Work out the finished part from the listing and answer in its coordinate system (mm). Face numbers are marked on the shaded views. A direction names the side the tool comes from. Round coordinates to 2 decimals unless told otherwise and drop trailing zeros. Order: outer loops, then holes, each group sorted by start corner. A loop starts at its lowest first (then second) coordinate and runs counter-clockwise, first axis right, second up. Notation, with made-up numbers: (28, -1.75) -> (52, -1.75) arc R26 cw to (52, 19.25) -> close; hole circle Ø3 at (-25, 74.25). An arc over 180 degrees is marked (long way). Use a Markdown table: item, result. Add a question column.
Item 1: Find the intervals of material crossed by L1, parallel to Y at x = -53, z = -21; L2, parallel to Z at x = -8.5, y = -10; L3, parallel to X at y = -12, z = 15, in increasing order. Write a range as [from, to].
Item 2: Flat-ended cylindrical pins translate along their axes: P1, Ø11.5, axis at y = -14.5, z = -6, coming from the -X side; P2, Ø1, axis at y = -14.5, z = 13.5, coming from the +X side; P3, Ø3, axis at y = -13, z = 2.5, coming from the +X side; P4, Ø6, axis at x = 6.5, y = -7.5, coming from the -Z side. Find the tip coordinate at first contact, or state that the pin passes through.
Item 3: A cutting plane is placed at D-D, the plane x = -24.5. Determine the outline of the cut face in (y, z).
Item 4: For a pull along Z with two mould halves and no side action, classify the marked faces 3, 4, 5 and 6 as +Z half, -Z half, draft (parallel to the pull), parting line (faces both ways), or undercut.
Item 5: A tool of negligible diameter and unlimited length cuts with its end or side. For the marked faces 1 and 2, from which of +Z, -Z, +X, -X, +Y, -Y can it reach the whole face along a straight path? Write none if from no direction.
Item 6: A cutting plane is placed at C-C, the plane y = -3. Determine the outline of the cut face in (x, z) (3 decimals).
Item 7: A cutting plane is placed at B-B, the plane z = 9. Determine the outline of the cut face in (x, y), plus the area to 3 significant figures.
Item 8: A cutting plane is placed at A-A, the plane y = -34. Determine the outline of the cut face in (x, z).
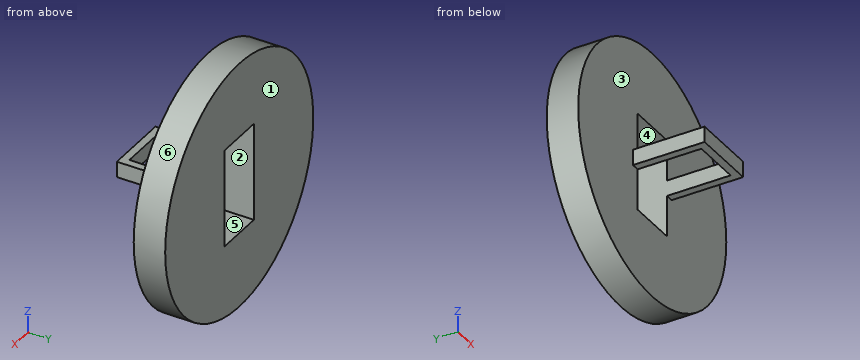
from build123d import *

# Parameters (mm, degrees)
F0_R     = 50.165
F0_W     = 19.812
F0_H     = 39.624
F1_DEPTH = 12.7
F3_DEPTH = 28.9052
F4_W     = 3.175
F4_H     = 6.35
F5_DEPTH = 19.812


with BuildPart() as f1:
    # F0 (on Front) → F1 (new body)
    with BuildSketch(Plane.XZ):
        with Locations((-8.635654, -2.157946)):
            Circle(F0_R)
        with Locations((-8.635654, -2.157946)):
            Rectangle(F0_W, F0_H, mode=Mode.SUBTRACT)
    extrude(amount=F1_DEPTH)

    # F2 (on face) → F3 (join)
    with BuildSketch(Plane.XZ.offset(12.7)):
        Polygon((-18.541654, -2.157946), (-18.541654, 1.017054), (-21.716654, 1.017054), (-21.716654, -2.157946), (-21.716654, -5.332946), (-18.541654, -5.332946), align=None)
        Polygon((4.445346, 1.017054), (1.270346, 1.017054), (1.270346, -2.157946), (1.270346, -5.332946), (4.445346, -5.332946), (4.445346, -2.157946), align=None)
    extrude(amount=F3_DEPTH)

    # F4 (on face) → F5 (join)
    with BuildSketch(Plane.YZ.offset(-18.541654)):
        with Locations((-40.0177, -2.157946)):
            Rectangle(F4_W, F4_H)
    extrude(amount=F5_DEPTH)


solid = f1.part
Reported:
| question | item | result |
|---|---|---|
| 1 | L1 | [-12.7, 0] |
| 1 | L2 | [-52.32, -21.97], [17.65, 48.01] |
| 1 | L3 | [-55.78, -18.54], [1.27, 38.5] |
| 2 | P1 | x = -58.8 |
| 2 | P2 | through |
| 2 | P3 | x = 41.43 |
| 2 | P4 | z = -50.83 |
| 3 | outline | (-12.7, -49.75) -> (0, -49.75) -> (0, 45.43) -> (-12.7, 45.43) -> close |
| 4 | face 3 | draft |
| 4 | face 4 | undercut |
| 4 | face 5 | undercut |
| 4 | face 6 | parting line |
| 5 | face 1 | +Z, -Z, +X, -X, +Y |
| 5 | face 2 | +Y |
| 6 | outline | circle Ø100.33 at (-8.636, -2.158); hole (-18.542, -21.97) -> (1.27, -21.97) -> (1.27, 17.654) -> (-18.542, 17.654) -> close |
| 7 | outline | (-57.54, -12.7) -> (-18.54, -12.7) -> (-18.54, 0) -> (-57.54, 0) -> close; (1.27, -12.7) -> (40.27, -12.7) -> (40.27, 0) -> (1.27, 0) -> close |
| 7 | area | 991 mm² |
| 8 | outline | (-21.72, -5.33) -> (-18.54, -5.33) -> (-18.54, 1.02) -> (-21.72, 1.02) -> close; (1.27, -5.33) -> (4.45, -5.33) -> (4.45, 1.02) -> (1.27, 1.02) -> close |
